from build123d import *

# Parameters (mm, degrees)
BOSS_EXTRUDE1_DEPTH = 5.4
BOSS_EXTRUDE2_DEPTH = 5.4


with BuildPart() as part:
    # Sketch1 → Boss-Extrude1 (new body)
    with BuildSketch(Plane.XY):
        Polygon((-239.303382108, -8.567555325), (-239.303382108, -13.967555325), (-244.703382108, -13.967555325), (-244.703382108, -62.232555325), (-239.303382108, -62.232555325), (-239.303382108, -110.497555325), (-244.703382108, -110.497555325), (-244.703382108, -158.762555325), (-239.303382108, -158.762555325), (-239.303382108, -207.027555325), (-244.703382108, -207.027555325), (-244.703382108, -255.292555325), (-224.878382108, -255.292555325), (-224.878382108, -207.027555325), (-219.478382108, -207.027555325), (-219.478382108, -158.762555325), (-224.878382108, -158.762555325), (-224.878382108, -110.497555325), (-219.478382108, -110.497555325), (-219.478382108, -62.232555325), (-224.878382108, -62.232555325), (-224.878382108, -8.567555325), align=None)
    extrude(amount=BOSS_EXTRUDE1_DEPTH)

    # Sketch2 → Boss-Extrude2 (add)
    with BuildSketch(Plane.XY.offset(5.4)):
        Polygon((-239.344022108, -8.526915325), (-239.344022108, -13.926915325), (-244.744022108, -13.926915325), (-244.744022108, -62.273195325), (-239.344022108, -62.273195325), (-239.344022108, -110.456915325), (-244.744022108, -110.456915325), (-244.744022108, -158.803195325), (-239.344022108, -158.803195325), (-239.344022108, -206.986915325), (-244.744022108, -206.986915325), (-244.744022108, -255.333195325), (-224.837742108, -255.333195325), (-224.837742108, -207.068195325), (-219.437742108, -207.068195325), (-219.437742108, -158.721915325), (-224.837742108, -158.721915325), (-224.837742108, -110.538195325), (-219.437742108, -110.538195325), (-219.437742108, -62.191915325), (-224.837742108, -62.191915325), (-224.837742108, -8.526915325), align=None)
    extrude(amount=-BOSS_EXTRUDE2_DEPTH)


solid = part.part
Model file for the job. Use its own axes, mm. A direction names the side the tool comes from. Give positions to 0.01 mm unless a question says otherwise; leave off trailing zeros. Loops run counter-clockwise (first coordinate to the right, second up) from the corner with the lowest first, then second, coordinate; pieces in that order, holes last. Notation, with made-up numbers: (-6, 19) -> (45, 19) arc R26 cw to (45, 35) -> close; hole circle Ø2 at (-23.75, 64.25). An arc over 180 degrees is marked (long way). Use a Markdown table: item, result. Add a question column.
(1) Slice it at B-B on z = 4.25. List the corners of the cut face in (x, y), and give its area (3 significant figures).
(2) Wall check: line 1 along Y through (x, z) = (-220.25, 2.6); line 2 along Y through (x, z) = (-241.75, 0.8); line 3 along X through (y, z) = (-49.5, 4.2). Give the ranges that are in metal, low to high.
(3) Mould opens along Y. For faces 5 (the flat face through (-222, -110.538, 3)), 6 (the flat face through (-224.838, -36, 3)), 7 (the flat face through (-222, -62.192, 3)), 8 (the flat face through (-222, -207.068, 3)) say: +Y half, -Y half, draft (parallel to the pull), parting line (faces both ways), or undercut.
(4) Slice it at A-A on x = -242.75. List the corners of the cut face in (y, z).
(5) Slice it at C-C on y = -45. List the corners of the cut face in (x, z), and give its area (3 significant figures).
(6) Tool access for faces 1 (the flat face through (-242, -158.803, 3)), 2 (the flat face through (-224.838, -135, 3)), 3 (the flat face through (-242, -13.927, 3)), 4 (the flat face through (-224.838, -232, 3)): list every direction of +Z, -Z, +X, -X, +Y, -Y with a clear straight run to the whole face (end or side of a thin tool).
(7) Drop flat-ended pins along their axis: pin 1 Ø2.5 at (x, z) = (-221.5, 1.5) entering from +Y; pin 2 Ø1.5 at (y, z) = (-89.5, 1.5) entering from -X. Give the stop position or say it passes through.
Filled sheet:
| question | item | result |
|---|---|---|
| 1 | outline | (-244.74, -255.33) -> (-224.84, -255.33) -> (-224.84, -207.07) -> (-219.44, -207.07) -> (-219.44, -158.72) -> (-224.84, -158.72) -> (-224.84, -110.54) -> (-219.44, -110.54) -> (-219.44, -62.19) -> (-224.84, -62.19) -> (-224.84, -8.53) -> (-239.34, -8.53) -> (-239.34, -13.93) -> (-244.74, -13.93) -> (-244.74, -62.27) -> (-239.34, -62.27) -> (-239.34, -110.46) -> (-244.74, -110.46) -> (-244.74, -158.8) -> (-239.34, -158.8) -> (-239.34, -206.99) -> (-244.74, -206.99) -> close |
| 1 | area | 4,890 mm2 |
| 2 | line 1 | -207.07 to -158.72, -110.54 to -62.19 |
| 2 | line 2 | -255.33 to -206.99, -158.8 to -110.46, -62.27 to -13.93 |
| 2 | line 3 | -244.74 to -224.84 |
| 3 | face 5 | undercut |
| 3 | face 6 | draft |
| 3 | face 7 | +Y half |
| 3 | face 8 | -Y half |
| 4 | outline | (-255.33, 0) -> (-206.99, 0) -> (-206.99, 5.4) -> (-255.33, 5.4) -> close; (-158.8, 0) -> (-110.46, 0) -> (-110.46, 5.4) -> (-158.8, 5.4) -> close; (-62.27, 0) -> (-13.93, 0) -> (-13.93, 5.4) -> (-62.27, 5.4) -> close |
| 5 | outline | (-244.74, 0) -> (-224.84, 0) -> (-224.84, 5.4) -> (-244.74, 5.4) -> close |
| 5 | area | 107 mm2 |
| 6 | face 1 | +Z, -Z, -X |
| 6 | face 2 | +Z, -Z, +X |
| 6 | face 3 | +Z, -Z, -X, +Y |
| 6 | face 4 | +Z, -Z, +X, -Y |
| 7 | pin 1 | y = -62.19 |
| 7 | pin 2 | x = -239.34 |
